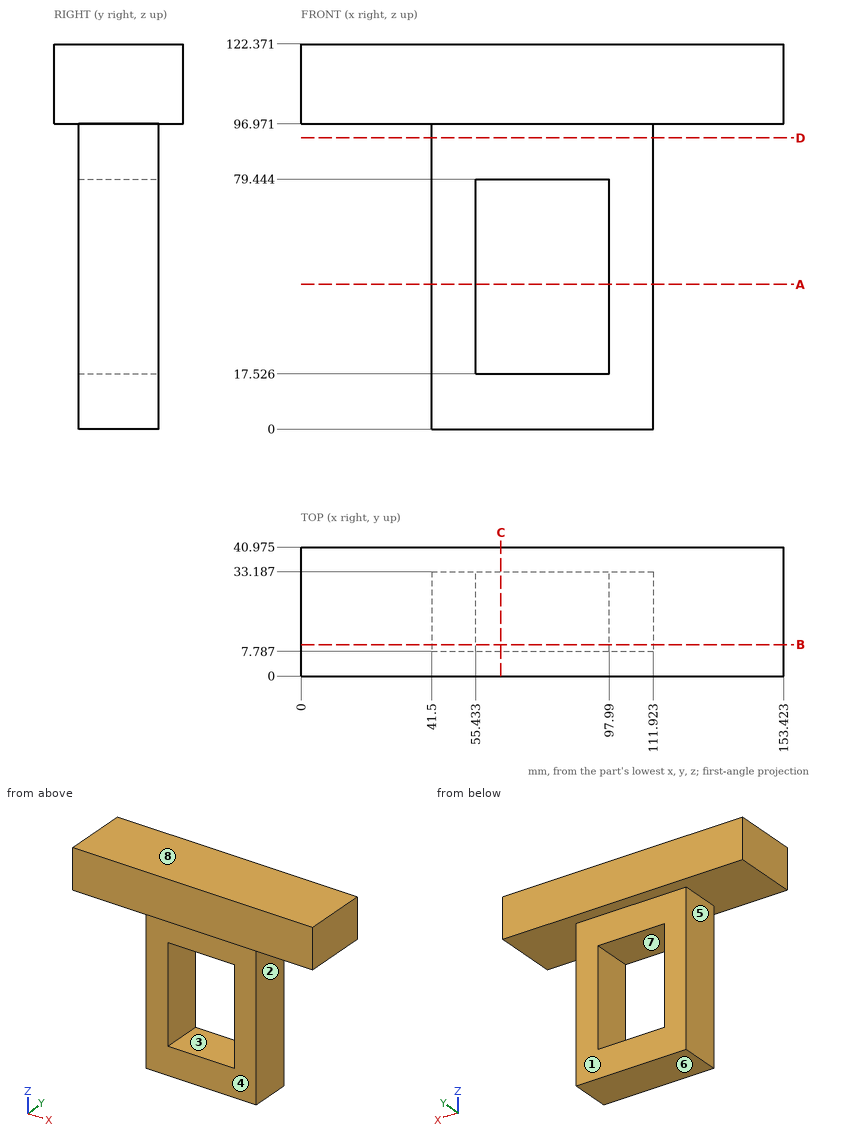
The figure shows three views and two pictorial views of one solid part (mm, origin at its lowest corner). Answer the questions. A direction names the side the tool comes from. Coordinates: 2 decimals unless noted, no trailing zeros. Loops run counter-clockwise (first coordinate to the right, second up) from the corner with the lowest first, then second, coordinate; pieces in that order, holes last.
1) Find the intervals of material crossed by L1, parallel to Z at x = 94, y = 16.5 (1 decimal); L2, parallel to X at y = 31, z = 61; L3, parallel to Z at x = 15, y = 21, in increasing order.
2) Flat-ended cylindrical pins translate along their axes: pin 1 Ø7.5 at (y, z) = (20, 37.5) entering from -X; pin 2 Ø10 at (y, z) = (7, 29) entering from +X; pin 3 Ø1.5 at (x, z) = (91.5, 84) entering from +Y. Find the tip coordinate at first contact, or state that the pin passes through.
3) Determine the mould class of the marked faces 5, 6, 7 and 8 for opening direction Z: pulls with the +Z half, pulls with the -Z half, needs draft (parallel to the pull), parting line crosses it, or undercut.
4) A tool of negligible diameter and unlimited length cuts with its end or side. For the marked faces 1, 2, 3 and 4, from which of +Z, -Z, +X, -X, +Y, -Y can it reach the whole face along a straight path? Write none if from no direction.
5) Find section D-D on z = 92.5. Write down the section's boundary in (x, y).
6) Find section C-C on x = 63.5. Write down the section's boundary in (y, z) (1 decimal).
7) Find section A-A on z = 46. Write down the section's boundary in (x, y).
8) Find section B-B on y = 10. Write down the section's boundary in (x, z) (1 decimal).
Values:
1. L1: z = 0 to 17.5, 79.4 to 122.4
1. L2: x = 41.5 to 55.43, 97.99 to 111.92
1. L3: z = 96.97 to 122.37
2. pin 1: stops at x = 41.5
2. pin 2: stops at x = 111.92
2. pin 3: stops at y = 33.19
3. face 5: needs draft
3. face 6: pulls with the -Z half
3. face 7: undercut
3. face 8: pulls with the +Z half
4. face 1: -Z, +X, -X, +Y
4. face 2: -Z, +X, +Y, -Y
4. face 3: +Y, -Y
4. face 4: -Z, +X, -X, -Y
5. outline: (41.5, 7.79) - (111.92, 7.79) - (111.92, 33.19) - (41.5, 33.19) - close
6. outline: (0, 97) - (7.8, 97) - (7.8, 79.4) - (33.2, 79.4) - (33.2, 97) - (41, 97) - (41, 122.4) - (0, 122.4) - close; (7.8, 0) - (33.2, 0) - (33.2, 17.5) - (7.8, 17.5) - close
7. outline: (41.5, 7.79) - (55.43, 7.79) - (55.43, 33.19) - (41.5, 33.19) - close; (97.99, 7.79) - (111.92, 7.79) - (111.92, 33.19) - (97.99, 33.19) - close
8. outline: (0, 97) - (41.5, 97) - (41.5, 0) - (111.9, 0) - (111.9, 97) - (153.4, 97) - (153.4, 122.4) - (0, 122.4) - close; hole (55.4, 17.5) - (98, 17.5) - (98, 79.4) - (55.4, 79.4) - close
